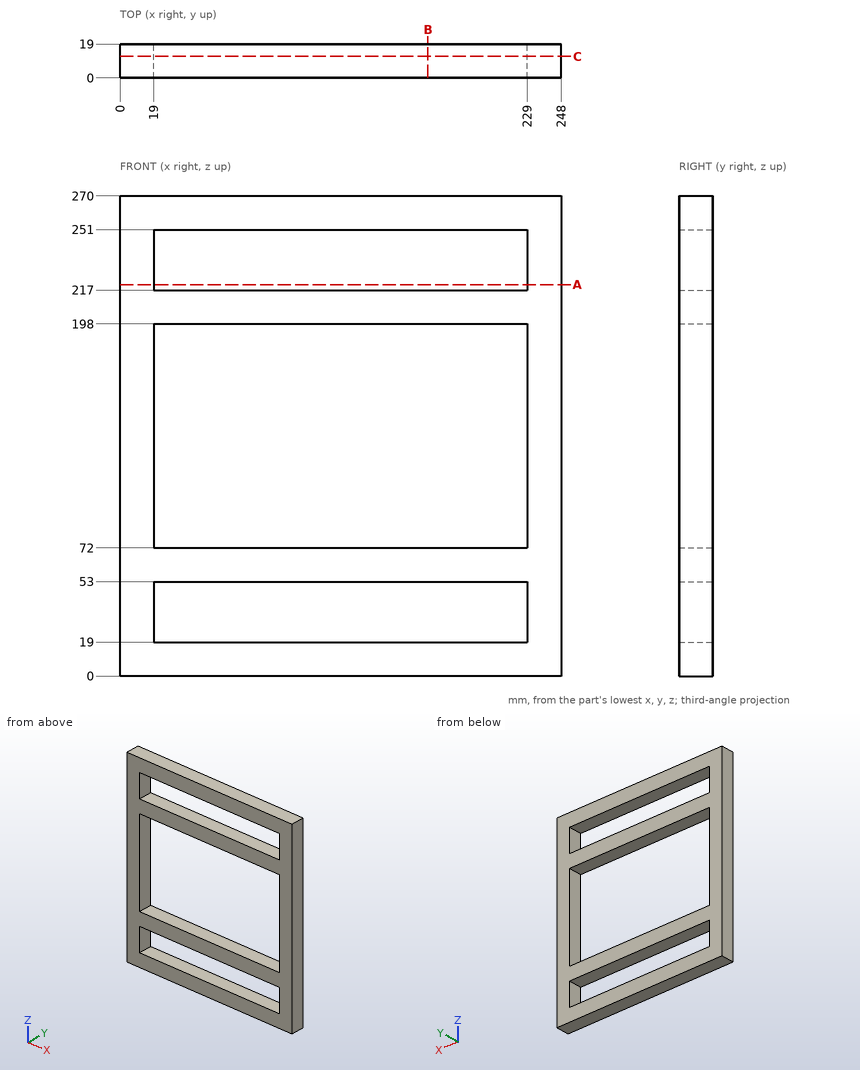
The figure shows three views and two pictorial views of one solid part (mm, origin at its lowest corner). Answer the questions. Round coordinates to 2 decimals unless told otherwise and drop trailing zeros. Loops run counter-clockwise (first coordinate to the right, second up) from the corner with the lowest first, then second, coordinate; pieces in that order, holes last. Notation, with made-up numbers: M 73,-32.75 L 125,-32.75 A20 cw 125,1.25 Z; hole C -27,-34 d4. An arc over 180 degrees is marked long. Return JSON: item names as keys, results as strings.
Q1. This flat-tipped pin is pushed along its axis until it touches: pin 1 Ø2 at (x, y) = (49, 9) entering from -Z. Where does it stop, or does it pass through?
Results list:
{"pin 1": "stops at z = 0"}
Q2. Find section C-C, the plane y = 12. Determine the outline of the cut face in (x, z).
Results list:
{"outline": "M 0,0 L 248,0 L 248,270 L 0,270 Z; hole M 19,19 L 229,19 L 229,53 L 19,53 Z; hole M 19,72 L 229,72 L 229,198 L 19,198 Z; hole M 19,217 L 229,217 L 229,251 L 19,251 Z"}
Q3. Find section A-A, the plane z = 220. Determine the outline of the cut face in (x, y).
Results list:
{"outline": "M 0,0 L 19,0 L 19,19 L 0,19 Z; M 229,0 L 248,0 L 248,19 L 229,19 Z"}
Q4. Find section B-B, the plane x = 173. Determine the outline of the cut face in (y, z), plus the area to 3 significant figures.
Results list:
{"outline": "M 0,0 L 19,0 L 19,19 L 0,19 Z; M 0,53 L 19,53 L 19,72 L 0,72 Z; M 0,198 L 19,198 L 19,217 L 0,217 Z; M 0,251 L 19,251 L 19,270 L 0,270 Z", "area": "1,440 mm2"}
Q5. Find the intervals of material crossed by line 1 along Z through (x, y) = (209, 7); line 2 along X through (y, z) = (16, 80), in increasing order. Write a range as from..to.
Results list:
{"line 1": "z = 0..19, 53..72, 198..217, 251..270", "line 2": "x = 0..19, 229..248"}
